Geometry: final body of the model. Coordinates: model frame, mm. A direction names the side the tool comes from. Give positions to 0.01 mm unless a question says otherwise; leave off trailing zeros. Order: outer loops, then holes, each group sorted by start corner. A loop starts at its lowest first (then second) coordinate and runs counter-clockwise, first axis right, second up. Notation, with made-up numbers: (-17.5, 44.5) - (9.5, 44.5) arc R23 cw to (9.5, 69.5) - close; hole circle Ø3 at (-23.5, 76). An arc over 180 degrees is marked (long way). Use one line per item in the form item = value.
Autodesk Inventor part; units mm, degrees
ref_plane "Work Plane1" through (0, 0, 0) normal (0, 0, 1) x (1, 0, 0)
ref_plane "YZ Plane" through (0, 0, 0) normal (1, 0, 0) x (0, 1, 0)
ref_plane "XZ Plane" through (0, 0, 0) normal (0, 1, 0) x (-1, 0, 0)
ref_plane "Work Plane1" through (0, 0, 0) normal (0, 0, 1) x (1, 0, 0)
sketch "Sketch1" plane through (0, 0, 0) normal (0, 0, 1) x (1, 0, 0)
  line L0 (-12.431, 44.25) -> (12.431, 44.25)
  line L1 (12.431, 44.25) -> (12.431, -44.25)
  line L2 (12.431, -44.25) -> (-12.431, -44.25)
  line L3 (-12.431, -44.25) -> (-12.431, 44.25)
  line L4 (-14.931, 46.75) -> (-14.931, -46.75)
  line L5 (-14.931, -46.75) -> (14.931, -46.75)
  line L6 (14.931, -46.75) -> (14.931, 46.75)
  line L7 (14.931, 46.75) -> (-14.931, 46.75)
  circle A0 centre (-9.931, -20.75) radius 1.1
  circle A1 centre (-9.931, -41.75) radius 1.1
  circle A2 centre (2.569, -41.75) radius 1.1
  circle A3 centre (2.569, -20.75) radius 1.1
  circle A4 centre (-9.931, 20.75) radius 1.1
  circle A5 centre (2.569, 20.75) radius 1.1
  circle A6 centre (-9.931, 41.75) radius 1.1
  circle A7 centre (2.569, 41.75) radius 1.1
  line L8 (6.4721, 35.2583) -> (-1.5279, 35.2583)
  line L9 (-1.5279, 35.2583) -> (-1.5279, 27.2583)
  line L10 (-1.5279, 27.2583) -> (6.4721, 27.2583)
  line L11 (6.4721, 27.2583) -> (6.4721, 35.2583)
  circle A8 centre (2.4721, 31.2583) radius 3.8
  line L12 (6.4721, -27.2417) -> (-1.5279, -27.2417)
  line L13 (-1.5279, -27.2417) -> (-1.5279, -35.2417)
  line L14 (-1.5279, -35.2417) -> (6.4721, -35.2417)
  line L15 (6.4721, -35.2417) -> (6.4721, -27.2417)
  circle A9 centre (2.4721, -31.2417) radius 3.8
  point P0 (0, 0)
extrude "Extrusion1" add sketch "Sketch1" along normal blind 2 contours L0 L1 L2 L3 | L7 L6 L5 L4
sketch "Sketch2" plane through (0, 0, 2) normal (0, 0, 1) x (1, 0, 0)
  line L0 (-1.5279, 27.2583) -> (6.4721, 27.2583)
  line L1 (-1.5279, 35.2583) -> (-1.5279, 27.2583)
  line L2 (6.4721, 35.2583) -> (-1.5279, 35.2583)
  line L3 (6.4721, 27.2583) -> (6.4721, 35.2583)
  line L4 (-1.5279, -27.2417) -> (-1.5279, -35.2417)
  line L5 (-1.5279, -35.2417) -> (6.4721, -35.2417)
  line L6 (6.4721, -27.2417) -> (-1.5279, -27.2417)
  line L7 (6.4721, -35.2417) -> (6.4721, -27.2417)
  line L8 (6.4721, -35.2417) -> (-1.5279, -35.2417)
  line L9 (-1.5279, -35.2417) -> (-1.5279, -35.4417)
  line L10 (-1.5279, -35.4417) -> (6.4721, -35.4417)
  line L11 (6.4721, -35.4417) -> (6.6721, -35.4417)
  line L12 (6.6721, -35.4417) -> (6.6721, -27.2417)
  line L13 (6.6721, -27.2417) -> (6.6721, -27.0417)
  line L14 (6.6721, -27.0417) -> (-1.5279, -27.0417)
  line L15 (-1.5279, -27.0417) -> (-1.7279, -27.0417)
  line L16 (-1.7279, -27.0417) -> (-1.7279, -35.4417)
  line L17 (-1.7279, -35.4417) -> (-1.5279, -35.4417)
  line L18 (6.4721, 35.2583) -> (6.4721, 27.2583)
  line L19 (6.4721, 27.2583) -> (6.6721, 27.2583)
  line L20 (6.6721, 27.2583) -> (6.6721, 35.2583)
  line L21 (6.6721, 35.2583) -> (6.6721, 35.4583)
  line L22 (6.6721, 35.4583) -> (-1.5279, 35.4583)
  line L23 (-1.5279, 35.4583) -> (-1.7279, 35.4583)
  line L24 (-1.7279, 35.4583) -> (-1.7279, 27.2583)
  line L25 (-1.7279, 27.2583) -> (-1.7279, 27.0583)
  line L26 (-1.7279, 27.0583) -> (6.6721, 27.0583)
  line L27 (6.6721, 27.0583) -> (6.6721, 27.2583)
  point P0 (0, 0)
  dimension "d2" = 0.2
  dimension "d3" = 0.2
  dimension "d4" = 0.2
  dimension "d5" = 0.2
  dimension "d6" = 0.2
  dimension "d7" = 0.2
  dimension "d8" = 0.2
  dimension "d9" = 0.2
extrude "Extrusion2" cut sketch "Sketch2" against normal through all
sketch "Sketch3" plane through (0, 0, 0) normal (0, 0, -1) x (-1, 0, 0)
  line L0 (12.431, 44.25) -> (-12.431, 44.25)
  line L1 (-12.431, 44.25) -> (-12.431, -44.25)
  line L2 (-12.431, -44.25) -> (12.431, -44.25)
  line L3 (12.431, -44.25) -> (12.431, 44.25)
  line L4 (14.931, 46.75) -> (14.931, -46.75)
  line L5 (14.931, -46.75) -> (-14.931, -46.75)
  line L6 (-14.931, -46.75) -> (-14.931, 46.75)
  line L7 (-14.931, 46.75) -> (14.931, 46.75)
  point P0 (0, 0)
extrude "Extrusion3" add sketch "Sketch3" along normal blind 3.05
sketch "Sketch4" plane through (0, 0, 2) normal (0, 0, 1) x (1, 0, 0)
  line L0 (6.6721, -35.4417) -> (-1.7279, -35.4417)
  line L1 (-1.7279, -35.4417) -> (-1.7279, -27.0417)
  line L2 (-1.7279, -27.0417) -> (6.6721, -27.0417)
  line L3 (6.6721, -27.0417) -> (6.6721, -35.4417)
  line L4 (-1.7279, 27.0583) -> (-1.7279, 35.4583)
  line L5 (6.6721, 27.0583) -> (-1.7279, 27.0583)
  line L6 (6.719, 35.5) -> (-1.781, 35.5)
  line L7 (6.6721, 35.4583) -> (6.6721, 27.0583)
  line L8 (6.6721, 27.0583) -> (6.6721, 35.4583)
  line L9 (6.6721, 31.2583) -> (2.4721, 31.2583)
  line L10 (-1.7279, 27.0583) -> (6.6721, 27.0583)
  line L11 (2.4721, 31.2583) -> (2.4721, 35.4583)
  line L12 (6.6721, 35.4583) -> (-1.7279, 35.4583)
  line L13 (6.6721, -31.2417) -> (2.4721, -31.2417)
  line L14 (2.4721, -31.2417) -> (2.4721, -27.0417)
  circle A0 centre (2.4721, 31.2583) radius 4.2
  circle A1 centre (2.4721, -31.2417) radius 4.2
  point P0 (0, 0)
  point P1 (2.4721, -35.4417)
  point P2 (-1.7279, -31.2417)
  point P3 (-1.7279, 31.2583)
  point P4 (2.4721, 27.0583)
extrude "Extrusion4" add sketch "Sketch4" against normal up to surface (2 mm away) contours L0 A1 L3 | L0 L1 A1 | A1 L2 L3 | L1 L2 A1 | L4 A0 L5 | L4 L12 A0 | A0 L7 L5 | L12 L7 A0
sketch "Sketch5" plane through (0, 0, 0) normal (0, 0, -1) x (-1, 0, 0)
  circle A0 centre (9.931, -20.75) radius 2
  circle A1 centre (9.931, -41.75) radius 2
  circle A2 centre (-2.569, -41.75) radius 2
  circle A3 centre (-2.569, -20.75) radius 2
  circle A4 centre (9.931, 20.75) radius 2
  circle A5 centre (-2.569, 20.75) radius 2
  circle A6 centre (9.931, 41.75) radius 2
  circle A7 centre (-2.569, 41.75) radius 2
  circle A8 centre (-2.569, 20.75) radius 1.1
  circle A9 centre (9.931, 20.75) radius 1.1
  circle A10 centre (9.931, 41.75) radius 1.1
  circle A11 centre (-2.569, 41.75) radius 1.1
  circle A12 centre (9.931, -20.75) radius 1.1
  circle A13 centre (-2.569, -20.75) radius 1.1
  circle A14 centre (-2.569, -41.75) radius 1.1
  circle A15 centre (9.931, -41.75) radius 1.1
  point P0 (0, 0)
extrude "Extrusion5" add sketch "Sketch5" along normal blind 3.05
sketch "Sketch6" plane through (0, 0, 2) normal (0, 0, 1) x (1, 0, 0)
  circle A0 centre (-9.931, -20.75) radius 1.1
  line L0 (-9.931, -20.75) -> (-9.931, 0)
  circle A1 centre (-9.931, 0) radius 1.45
  circle A2 centre (2.569, 0) radius 1.45
  circle A3 centre (-9.931, 0) radius 3
  circle A4 centre (2.569, 0) radius 3
  point P0 (0, 0)
  dimension "d18" = 20.75
  dimension "d19" = 2.9
  dimension "d20" = 2.9
  dimension "d21" = 6
  dimension "d22" = 6
extrude "Extrusion6" cut sketch "Sketch6" against normal through all contours A1 | A2
extrude "Extrusion7" add sketch "Sketch6" against normal up to surface (5.05 mm away) contours A3 | A4
sketch "Sketch7" plane through (0, 0, 2) normal (0, 0, 1) x (1, 0, 0)
  circle A0 centre (2.569, 20.75) radius 1.1
  circle A1 centre (-9.931, 20.75) radius 1.1
  circle A2 centre (2.569, 41.75) radius 1.1
  circle A3 centre (-9.931, 41.75) radius 1.1
  circle A4 centre (2.569, -20.75) radius 1.1
  circle A5 centre (2.569, -41.75) radius 1.1
  circle A6 centre (-9.931, -41.75) radius 1.1
  circle A7 centre (-9.931, -20.75) radius 1.1
  point P0 (0, 0)
extrude "Extrusion8" add sketch "Sketch7" against normal up to surface (5.05 mm away)
sketch "Sketch8" plane through (2.569, -41.75, -3.05) normal (0, 0, -1) x (-1, 0, 0)
  circle A0 centre (0, 0) radius 2
  circle A1 centre (0, 0) radius 0.8
  circle A2 centre (12.5, 0) radius 2
  circle A3 centre (12.5, 0) radius 0.8
  circle A4 centre (12.5, 21) radius 2
  circle A5 centre (12.5, 21) radius 0.8
  circle A6 centre (0, 21) radius 2
  circle A7 centre (0, 21) radius 0.8
  circle A8 centre (0, 62.5) radius 2
  circle A9 centre (0, 62.5) radius 0.8
  circle A10 centre (12.5, 62.5) radius 2
  circle A11 centre (12.5, 62.5) radius 0.8
  circle A12 centre (12.5, 83.5) radius 2
  circle A13 centre (12.5, 83.5) radius 0.8
  circle A14 centre (0, 83.5) radius 2
  circle A15 centre (0, 83.5) radius 0.8
  point P0 (2.569, 41.75)
  dimension "d29" = 1.6
  dimension "d30" = 1.6
  dimension "d31" = 1.6
  dimension "d32" = 1.6
  dimension "d33" = 1.6
  dimension "d34" = 1.6
  dimension "d35" = 1.6
  dimension "d36" = 1.6
extrude "Extrusion9" add sketch "Sketch8" along normal blind 1 contours A1 | A3 | A5 | A7 | A9 | A11 | A13 | A15
sketch "Sketch9" plane through (0, 0, 2) normal (0, 0, 1) x (1, 0, 0)
  circle A0 centre (-9.931, -50.25) radius 1.45
  circle A1 centre (2.473, -50.25) radius 1.45
  circle A2 centre (-9.931, 50.25) radius 1.45
  circle A3 centre (2.473, 50.25) radius 1.45
  line L0 (-12.431, 44.25) -> (12.431, 44.25)
  line L1 (12.431, 44.25) -> (12.431, -44.25)
  line L2 (12.431, -44.25) -> (-12.431, -44.25)
  line L3 (-12.431, -44.25) -> (-12.431, 44.25)
  line L4 (-14.931, -53.75) -> (-14.931, 53.75)
  line L5 (14.931, -53.75) -> (-14.931, -53.75)
  line L6 (14.931, 53.75) -> (14.931, -53.75)
  line L7 (-14.931, 53.75) -> (14.931, 53.75)
  point P0 (0, 0)
extrude "Extrusion10" add sketch "Sketch9" against normal up to surface (5.05 mm away)
properties part number "pi_cam_stereo_case_cover"
(1) Cut plane A-A on z = -1.5. Give the number of separate pieces and of enclosed holes in the cut face, plus the area to 3 significant figures.
Computed values:
separate_pieces = 10
enclosed_holes = 7
area = 1,130 mm²
(2) Cut plane D-D on y = 15. Output: boundary loops of the cut face in (x, z).
Computed values:
outline = (-14.93, -3.05) - (-12.43, -3.05) - (-12.43, 0) - (12.43, 0) - (12.43, -3.05) - (14.93, -3.05) - (14.93, 2) - (-14.93, 2) - close
(3) Reachability of faces 1 (the face through (-8.592, 49.695, -0.49)), 2 (the face through (-3, 1, 0)), 3 (the face through (4, 1, -3.05)) from +Z, -Z, +X, -X, +Y, -Y: full face, straight path, thin tool, end or side. Return the list, or none.
Computed values:
face_1 = +Z, -Z
face_2 = -Z
face_3 = -Z, +X, -X
(4) Ray query, line 1 along X through (y, z) = (-20.5, -1); line 2 along Y through (x, z) = (-3.75, -1.25); line 3 along X through (y, z) = (-37, -0.25). Return the intervals inside material, ascending.
Computed values:
line_1 = -14.93 to -12.43, -11.92 to -7.95, 0.58 to 4.55, 12.43 to 14.93
line_2 = -53.75 to -44.25, 44.25 to 53.75
line_3 = -14.93 to -12.43, 12.43 to 14.93
(5) Cut plane C-C on x = -5.5. Output: boundary loops of the cut face in (y, z), plus the area to 3 significant figures.
Computed values:
outline = (-53.75, -3.05) - (-44.25, -3.05) - (-44.25, 0) - (44.25, 0) - (44.25, -3.05) - (53.75, -3.05) - (53.75, 2) - (-53.75, 2) - close
area = 273 mm²
(6) Cut plane B-B on y = -50.25. Output: boundary loops of the cut face in (x, z).
Computed values:
outline = (-14.93, -3.05) - (-11.38, -3.05) - (-11.38, 2) - (-14.93, 2) - close; (-8.48, -3.05) - (1.02, -3.05) - (1.02, 2) - (-8.48, 2) - close; (3.92, -3.05) - (14.93, -3.05) - (14.93, 2) - (3.92, 2) - close
(7) Contact query for flat-ended pins moving along their axis: pin 1 Ø3 at (x, y) = (3.5, 41) entering from -Z; pin 2 Ø10 at (x, y) = (3.5, -10) entering from -Z; pin 3 Ø12 at (x, y) = (-3.5, 24.5) entering from -Z; pin 4 Ø5 at (x, y) = (2.47, -31.24) entering from +Z. Output: stop coordinate, or through.
Computed values:
pin_1 = -4.05
pin_2 = 0
pin_3 = -3.05
pin_4 = through
(8) Pull-direction query (X, two-part tool) for faces 4 (the face through (14.931, 1, 0)), 5 (the face through (0, -53.75, 0)), 6 (the face through (-9.671, -22.733, -1.504)), 7 (the face through (-9.262, -51.536, -0.49)); classes: released by +X, released by -X, zero draft, split by the parting line, or undercut.
Computed values:
face_4 = released by +X
face_5 = zero draft
face_6 = undercut
face_7 = undercut
